from build123d import *

# Parameters (mm, degrees)
BOSS_EXTRUDE1_DEPTH = 100
SKETCH3_W           = 7.7
SKETCH3_H           = 7.5
CUT_EXTRUDE1_DEPTH  = 207.039437972
SKETCH6_W           = 45.2
SKETCH6_H           = 15.4
CUT_EXTRUDE2_DEPTH  = 112.589650058


with BuildPart() as part:
    # Sketch1 → Boss-Extrude1 (new, symmetric)
    with BuildSketch(Plane(origin=(0, 0, 0), x_dir=(0, 0, -1), z_dir=(1, 0, 0))):
        Polygon((-48.5, 0), (48.5, 10), (48.5, 0), align=None)
    extrude(amount=BOSS_EXTRUDE1_DEPTH, both=True)

    # Sketch3 → Cut-Extrude1 (cut, through all)
    with BuildSketch(Plane(origin=(100, 0, 0), x_dir=(0, 0, -1), z_dir=(1, 0, 0))):
        with Locations((44.65, 3.75)):
            Rectangle(SKETCH3_W, SKETCH3_H)
    extrude(amount=-CUT_EXTRUDE1_DEPTH, mode=Mode.SUBTRACT)

    # Sketch6 → Cut-Extrude2 (cut, through all)
    with BuildSketch(Plane(origin=(0, 0, 0), x_dir=(1, 0, 0), z_dir=(0, 1, 0))):
        with Locations((77.4, 19)):
            Rectangle(SKETCH6_W, SKETCH6_H)
    extrude(amount=CUT_EXTRUDE2_DEPTH, mode=Mode.SUBTRACT)


solid = part.part
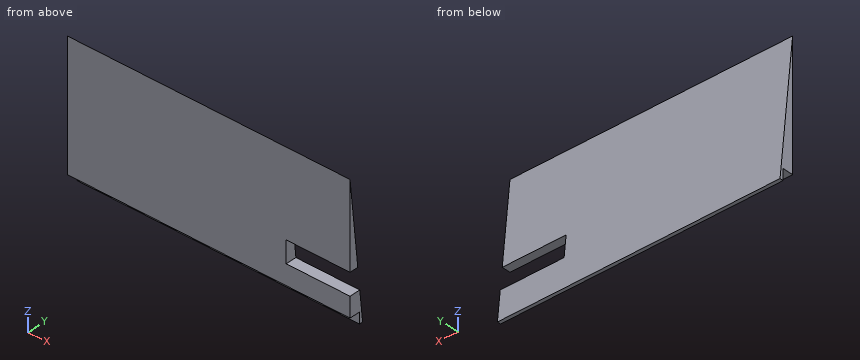
Verification items for the finished model (mm, model axes). Round coordinates to 2 decimals unless told otherwise and drop trailing zeros. Loops run counter-clockwise (first coordinate to the right, second up) from the corner with the lowest first, then second, coordinate; pieces in that order, holes last. Notation, with made-up numbers: (34, 28.5) - (38, 28.5) arc R28 cw to (38, 58.5) - close; hole circle Ø5 at (42.5, 71). An arc over 180 degrees is marked (long way). Use one line per item in the form item = value.
1. Section check B-B on y = 3.5. Record the cut outline in (x, z).
A:
outline = (-100, -40.8) - (100, -40.8) - (100, -26.7) - (54.8, -26.7) - (54.8, -11.3) - (100, -11.3) - (100, 14.55) - (-100, 14.55) - close
2. Scan lines: probe 1 along X at (y, z) = (5.5, -17.5); probe 2 along Y at (x, z) = (31, 18); probe 3 along Y at (x, z) = (-7.5, -42.5). Record each from-to range of solid material in increasing order.
A:
probe_1 = -100 to 54.8
probe_2 = 0 to 3.14
probe_3 = 7.5 to 9.38
3. Section check A-A on x = 62. Record the cut outline in (y, z).
A:
outline = (0, -40.8) - (7.5, -40.8) - (7.5, -48.5) - (10, -48.5) - (7.75, -26.7) - (0, -26.7) - close; (0, -11.3) - (6.16, -11.3) - (0, 48.5) - close
4. Section check D-D on z = 1. Record the cut outline in (x, y).
A:
outline = (-100, 0) - (100, 0) - (100, 4.9) - (-100, 4.9) - close
5. Section check C-C on x = -79.5. Record the cut outline in (y, z).
A:
outline = (0, -40.8) - (7.5, -40.8) - (7.5, -48.5) - (10, -48.5) - (0, 48.5) - close
6. Gauge pin test, flat ends, axial feed: pin 1 Ø2.5 at (x, z) = (-17, -44.5) entering from -Y; pin 2 Ø5 at (y, z) = (5, 11) entering from -X; pin 3 Ø1.5 at (x, y) = (70, 5) entering from -Z; pin 4 Ø6 at (y, z) = (2.5, -22.5) entering from +X. Record the tip position at first contact, or that the pin passes through.
A:
pin_1 = 7.5
pin_2 = -100
pin_3 = -40.8
pin_4 = 54.8
